CAD build for the part. Positions are in the model's coordinates, mm. Face numbers are marked on the shaded views. A direction names the side the tool comes from. Coordinates: 2 decimals unless noted, no trailing zeros. Write each loop counter-clockwise with the first axis right and the second up, starting at its lowest first coordinate (ties: lowest second). Pieces come first, ordered by that corner, then holes. Notation, with made-up numbers: M 51.5,-5 L 71.5,-5 A30 cw 71.5,29 Z; hole C 48,80.25 d3. An arc over 180 degrees is marked long. Answer as CSV lines item,"result". Start each with the question number.
```python
from build123d import *

# Parameters (mm, degrees)
BOSS_EXTRUDE1_DEPTH      = 32.31
CUT_EXTRUDE1_DEPTH       = 25
SKETCH3_W                = 3.5
SKETCH3_H                = 16.162716407
CUT_EXTRUDE2_DEPTH       = 16
SKETCH4_W                = 3
SKETCH4_H                = 8
BOSS_EXTRUDE2_DEPTH      = 32.31
FILLET1_R                = 1
FILLET2_R                = 1
M3_CLEARANCE_HOLE1_D     = 3.6
M3_CLEARANCE_HOLE1_DEPTH = 16
M3_CLEARANCE_HOLE1_TIP   = 1.081549114
CUT_EXTRUDE3_DEPTH       = 4


with BuildPart() as part:
    # Sketch1 → Boss-Extrude1 (new body)
    with BuildSketch(Plane(origin=(0, 0, 0), x_dir=(1, 0, 0), z_dir=(0, 1, 0))):
        with BuildLine():
            Line((-45, 13.25), (-25.841229183, 13.25))
            ThreePointArc((-25.841229183, 13.25), (-21, 17), (-16.158770817, 13.25))
            Line((-16.158770817, 13.25), (16.158770817, 13.25))
            ThreePointArc((16.158770817, 13.25), (21, 17), (25.841229183, 13.25))
            Line((25.841229183, 13.25), (45, 13.25))
            Line((45, 13.25), (45, 10.75))
            Line((45, 10.75), (25.841229183, 10.75))
            ThreePointArc((25.841229183, 10.75), (21, 7), (16.158770817, 10.75))
            Line((16.158770817, 10.75), (-16.158770817, 10.75))
            ThreePointArc((-16.158770817, 10.75), (-21, 7), (-25.841229183, 10.75))
            Line((-25.841229183, 10.75), (-45, 10.75))
            Line((-45, 10.75), (-45, 13.25))
        make_face()
    extrude(amount=BOSS_EXTRUDE1_DEPTH)

    # Sketch2 → Cut-Extrude1 (cut)
    with BuildSketch(Plane.XY.offset(-10.75)):
        Polygon((-35.420614591, 0), (-45, 26.272359302), (-58.390365854, 22.525370437), (-53.81468831, -5.500654521), (-35.420614591, -4.763359631), align=None)
        Polygon((53.81468831, -5.500654521), (35.420614591, -4.763359631), (35.420614591, 0), (45, 26.272359302), (58.390365854, 22.525370437), align=None)
    extrude(amount=-CUT_EXTRUDE1_DEPTH, mode=Mode.SUBTRACT)

    # Sketch3 → Cut-Extrude2 (cut)
    with BuildSketch(Plane(origin=(0, 32.31, 0), x_dir=(1, 0, 0), z_dir=(0, 1, 0))):
        with Locations((-28.25, 12.031966157)):
            Rectangle(SKETCH3_W, SKETCH3_H)
        with Locations((28.25, 12.031966157)):
            Rectangle(SKETCH3_W, SKETCH3_H)
    extrude(amount=-CUT_EXTRUDE2_DEPTH, mode=Mode.SUBTRACT)

    # Sketch4 → Boss-Extrude2 (add)
    with BuildSketch(Plane.XZ):
        with Locations((-31.5, -12)):
            Rectangle(SKETCH4_W, SKETCH4_H)
    boss_extrude2 = extrude(amount=-BOSS_EXTRUDE2_DEPTH)

    # Fillet1
    fillet1_edges = [part.edges().sort_by_distance(p)[0] for p in [
        (-33, 16.155, -10.75),
        (-33, 16.155, -8),
        (-33, 16.155, -13.25),
        (-33, 16.155, -16),
    ]]
    fillet(fillet1_edges, radius=FILLET1_R)

    # Mirror1: Boss-Extrude2 across plane
    add(boss_extrude2.mirror(Plane(origin=(0, 0, 0), x_dir=(0, 0, 1), z_dir=(1, 0, 0))))

    # Fillet2
    fillet2_edges = [part.edges().sort_by_distance(p)[0] for p in [
        (33, 16.155, -10.75),
        (33, 16.155, -8),
        (33, 16.155, -13.25),
        (33, 16.155, -16),
    ]]
    fillet(fillet2_edges, radius=FILLET2_R)

    # M3 Clearance Hole1
    with Locations(Plane(origin=(0, 0, 0), x_dir=(-1, 0, 0), z_dir=(0, -1, 0))):
        with Locations((-21, 12), (21, 12)):
            Hole(M3_CLEARANCE_HOLE1_D / 2, depth=M3_CLEARANCE_HOLE1_DEPTH)
            with Locations((0, 0, -(M3_CLEARANCE_HOLE1_DEPTH + M3_CLEARANCE_HOLE1_TIP / 2))):  # 118° drill point
                Cone(0, M3_CLEARANCE_HOLE1_D / 2, M3_CLEARANCE_HOLE1_TIP, mode=Mode.SUBTRACT)

    # Sketch7 → Cut-Extrude3 (cut)
    with BuildSketch(Plane(origin=(0, 10, 0), x_dir=(-1, 0, 0), z_dir=(0, -1, 0))):
        Polygon((-24.15, 13.818653348), (-24.15, 10.181346652), (-21, 8.362693304), (-17.85, 10.181346652), (-17.85, 13.818653348), (-17.85, 20.157444089), (-24.15, 20.157444089), align=None)
    cut_extrude3 = extrude(amount=CUT_EXTRUDE3_DEPTH, mode=Mode.SUBTRACT)

    # Mirror2: Cut-Extrude3 across plane
    add(cut_extrude3.mirror(Plane(origin=(0, 0, 0), x_dir=(0, 0, 1), z_dir=(1, 0, 0))), mode=Mode.SUBTRACT)


solid = part.part
```
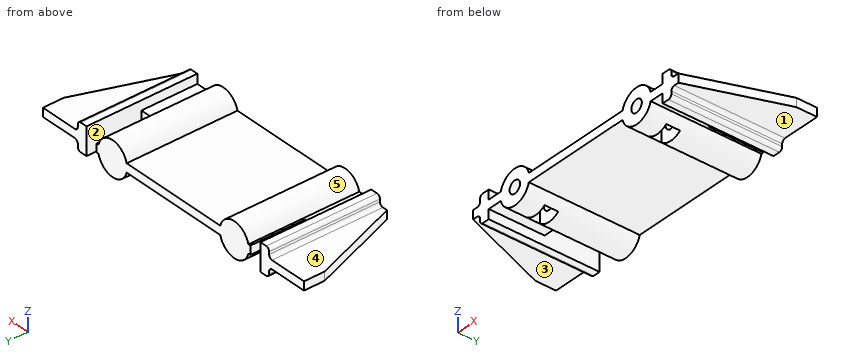
1) Tool access for the marked faces 1, 2 and 3: list every direction of +Z, -Z, +X, -X, +Y, -Y with a clear straight run to the whole face (end or side of a thin tool).
2) Pin check, flat tips, straight feed: P1, Ø1.9, axis at x = -21.5, z = -13.5, coming from the -Y side; P2, Ø5, axis at y = 17.5, z = -9, coming from the -X side; P3, Ø1.6, axis at x = -31.5, y = 15.5, coming from the -Z side; P4, Ø0.8, axis at y = 11, z = -14.5, coming from the -X side. Stop position of each tip, or through.
3) Band-saw the part on B-B, the plane x = -4.5. List the corners of the cut face in (y, z), plus the area to 3 significant figures.
4) Band-saw the part on C-C, the plane x = 38. List the corners of the cut face in (y, z), plus the area to 3 significant figures.
5) Probe L1, parallel to Z at x = -21, y = 13.5; L2, parallel to Y at x = 19, z = -11.75; L3, parallel to X at y = 27.5, z = -13. List the from-to ranges inside material, lowest first. Write a range as [from, to].
6) Band-saw the part on A-A, the plane y = 21. State how many separate pieces and enclosed holes the cut face has, plus the area to 3 significant figures.
7) Two-plate mould, pull along X, no slides. Class the marked faces 4 and 5: pulls with the +X half, pulls with the -X half, needs draft (parallel to the pull), parting line crosses it, or undercut.
Result sheet:
1,face 1,"-Z, +X, +Y, -Y"
1,face 2,"+Y"
1,face 3,"-Z, -X, +Y, -Y"
2,P1,"stops at y = 0"
2,P2,"stops at x = -42.45"
2,P3,"stops at z = -16"
2,P4,"stops at x = -33.01"
3,outline,"M 0,-13.25 L 32.31,-13.25 L 32.31,-10.75 L 0,-10.75 Z"
3,area,"80.8 mm²"
4,outline,"M 7.07,-13.25 L 32.31,-13.25 L 32.31,-10.75 L 7.07,-10.75 Z"
4,area,"63.1 mm²"
5,L1,"z = [-17, -13.8], [-10.2, -7]"
5,L2,"y = [0, 6], [10, 32.31]"
5,L3,"x = [-45, -30], [-26.5, 26.5], [30, 45]"
6,separate pieces,"3"
6,enclosed holes,"0"
6,area,"338 mm²"
7,face 4,"needs draft"
7,face 5,"undercut"
